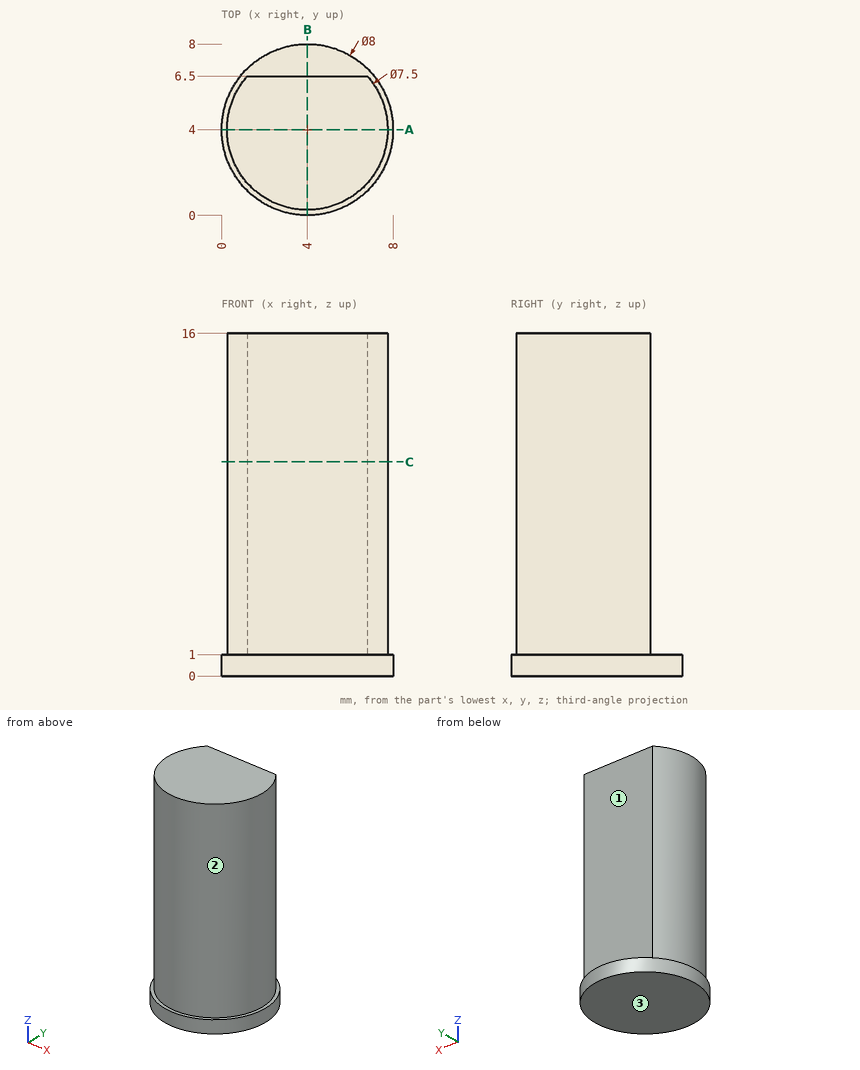
For this review, use the dimensioned drawing (mm, ordinates from the lowest corner) and the shaded views. A direction names the side the tool comes from. Give positions to 0.01 mm unless a question says otherwise; leave off trailing zeros. Order: outer loops, then holes, each group sorted by start corner. A loop starts at its lowest first (then second) coordinate and runs counter-clockwise, first axis right, second up.
1. Tool access review of the marked faces 1, 2 and 3: name each direction out of +Z, -Z, +X, -X, +Y, -Y from which nothing blocks a thin tool from reaching the whole face with its end or side.
Solution:
face 1: +Z, +X, -X, +Y
face 2: +Z
face 3: -Z, +X, -X, +Y, -Y
2. Add section A-A, the plane y = 4. State the section outline as (x, z) points, then the cut area to 4 significant figures.
Solution:
outline: (0, 0) - (8, 0) - (8, 1) - (7.75, 1) - (7.75, 16) - (0.25, 16) - (0.25, 1) - (0, 1) - close
area: 120.5 mm2
3. For pin 1 Ø4 at (y, z) = (1.5, 14.5) entering from +X; pin 2 Ø1 at (x, y) = (7, 5) entering from -Z; pin 3 Ø1 at (x, z) = (4.5, 13) entering from -Y, all flat-tipped, find the tip position at first contact; note any pin that passes through.
Solution:
pin 1: stops at x = 7.72
pin 2: stops at z = 0
pin 3: stops at y = 0.25
4. To check wall thickness, follow L1, parallel to Z at x = 3, y = 7.75; L2, parallel to X at y = 1.5, z = 13.5; L3, parallel to Y at x = 7.25, z = 6.25. State the ranges of each line that lie inside material, in increasing order.
Solution:
L1: z = 0 to 1
L2: x = 1.2 to 6.8
L3: y = 2.13 to 5.87
5. Add section B-B, the plane x = 4. State the section outline as (y, z) points, then the cut area to 3 significant figures.
Solution:
outline: (0, 0) - (8, 0) - (8, 1) - (6.5, 1) - (6.5, 16) - (0.25, 16) - (0.25, 1) - (0, 1) - close
area: 102 mm2
6. Add section C-C, the plane z = 10. State the section outline as (x, y) points, then the cut area to 3 significant figures.
Solution:
outline: (1.2, 6.5) arc R3.75 ccw (long way) to (6.8, 6.5) - close
area: 39.3 mm2
